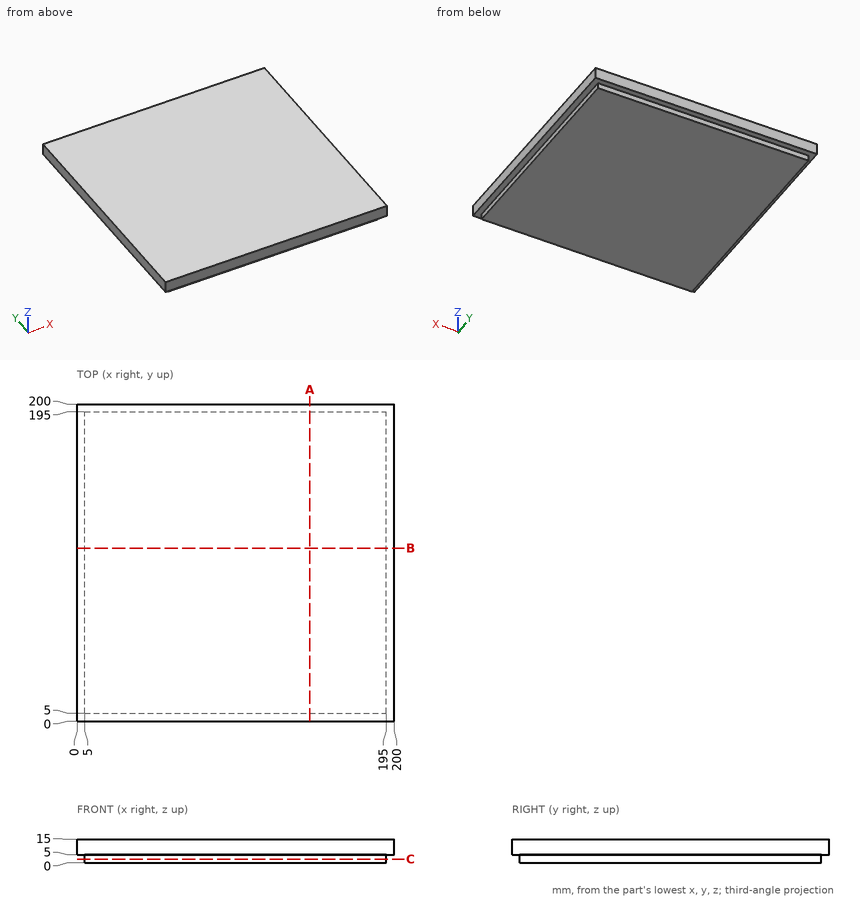
Job drawing, mm, ordinate dimensions from the low corner. One solid piece. Round coordinates to 2 decimals unless told otherwise and drop trailing zeros. Loops run counter-clockwise (first coordinate to the right, second up) from the corner with the lowest first, then second, coordinate; pieces in that order, holes last.
Item 1: Cut at A-A, the plane x = 147. Give the cut face in (y, z), then the cut area to 3 significant figures.
Item 2: Drill centre line: line 1 (Y direction, x = 84.5, z = 3.75). Where is it in solid material? Low to high.
Item 3: Drop flat-ended pins along their axis: P1, Ø5.5, axis at x = 113, z = 1.5, coming from the +Y side; P2, Ø5.5, axis at y = 63, z = 2, coming from the -X side; P3, Ø2.5, axis at y = 133.5, z = 1.5, coming from the +X side. Give the stop position or say it passes through.
Item 4: Cut at C-C, the plane z = 2.25. Give the cut face in (x, y), then the cut area to 3 significant figures.
A:
1. outline: (0, 5) - (5, 5) - (5, 0) - (195, 0) - (195, 5) - (200, 5) - (200, 15) - (0, 15) - close
1. area: 2,950 mm2
2. line 1: y = 5 to 195
3. P1: stops at y = 195
3. P2: stops at x = 5
3. P3: stops at x = 195
4. outline: (5, 5) - (195, 5) - (195, 195) - (5, 195) - close
4. area: 36,100 mm2
